from build123d import *

# Parameters (mm, degrees)
F0_W     = 50
F0_H     = 25
F1_DEPTH = 25
F2_R     = 4
F3_R     = 11
F4_DEPTH = 25.001


with BuildPart() as f1:
    # F0 (on Front) → F1 (new body, symmetric)
    with BuildSketch(Plane.XZ):
        with Locations((1, -12.5)):
            Rectangle(F0_W, F0_H)
    extrude(amount=F1_DEPTH, both=True)

    # F2
    f2_edges = [f1.edges().sort_by_distance(p)[0] for p in [
        (-24, 0, 0),
    ]]
    fillet(f2_edges, radius=F2_R)

    # F3 (on face) → F4 (cut, through all)
    with BuildSketch(Plane.XY):
        Circle(F3_R)
    extrude(amount=-F4_DEPTH, mode=Mode.SUBTRACT)


solid = f1.part
The model under review builds one solid part; all positions refer to its coordinate system, in mm. Round coordinates to 2 decimals unless told otherwise and drop trailing zeros. Write each loop counter-clockwise with the first axis right and the second up, starting at its lowest first coordinate (ties: lowest second). Pieces come first, ordered by that corner, then holes. Notation, with made-up numbers: M 62,-34.5 L 118,-34.5 A16 ccw 118,-23.5 Z; hole C -21.75,1 d10. An arc over 180 degrees is marked long. Answer as CSV lines item,"result". Start each with the question number.
Q1. The part is to be moulded in two halves that separate along Y. For faces 1 (the face through (-2.38, -10.74, -12.32)), 2 (the face through (1, -25, -12)), 3 (the face through (26, 0, -13)), say which applies: +Y half, -Y half, draft (parallel to the pull), parting line (faces both ways), or undercut.
Q2. Consider section B-B, the plane y = 0. Give the boundary of the cut face in (x, z).
Q3. Consider section A-A, the plane x = 0. Give the boundary of the cut face in (y, z).
Q4. Consider section D-D, the plane y = 9.5. Give the boundary of the cut face in (x, z).
Q5. Consider section C-C, the plane z = -7.5. Give the boundary of the cut face in (x, y), then the cut area to 3 significant figures.
Q6. Clearance check with a flat-ended pin moving along its axis: P1, Ø17.5, axis at x = 0, y = 0, coming from the -Z side. State where the tip first meets the part, or that it passes through.
Q7. Wall thickness on line 1 along Y through (x, z) = (0, -7.75); line 2 along X through (y, z) = (-9.5, -16.5); line 3 along X through (y, z) = (1, -9.75): over which ranges is each line inside the solid? List them lowest first.
Result set:
1,face 1,"undercut"
1,face 2,"-Y half"
1,face 3,"draft"
2,outline,"M -24,-25 L -11,-25 L -11,0 L -20,0 A4 ccw -24,-4 Z; M 11,-25 L 26,-25 L 26,0 L 11,0 Z"
3,outline,"M -25,-25 L -11,-25 L -11,0 L -25,0 Z; M 11,-25 L 25,-25 L 25,0 L 11,0 Z"
4,outline,"M -24,-25 L -5.55,-25 L -5.55,0 L -20,0 A4 ccw -24,-4 Z; M 5.55,-25 L 26,-25 L 26,0 L 5.55,0 Z"
5,outline,"M -24,-25 L 26,-25 L 26,25 L -24,25 Z; hole C 0,0 d22"
5,area,"2,120 mm²"
6,P1,"passes through"
7,line 1,"y = -25 to -11, 11 to 25"
7,line 2,"x = -24 to -5.55, 5.55 to 26"
7,line 3,"x = -24 to -10.95, 10.95 to 26"
